The listing builds one solid part. Answer for the finished solid, in the listing's coordinates (mm). Face numbers are marked on the shaded views. A direction names the side the tool comes from. Coordinates: 2 decimals unless noted, no trailing zeros. Write each loop counter-clockwise with the first axis right and the second up, starting at its lowest first coordinate (ties: lowest second). Pieces come first, ordered by that corner, then holes.
from build123d import *

# Parameters (mm, degrees)
F0_R     = 14.2875
F1_DEPTH = 25.4
F2_DEPTH = 50.8


# Not quite as in the source:
# - a fillet or chamfer that OpenCascade refuses, or shapes differently, is made with other operations: its cross-section is extruded or revolved along the edge and cut away or added


with BuildPart() as f1:
    # F0 (on Top) → F1 (new body)
    with BuildSketch(Plane.XY):
        with BuildLine():
            ThreePointArc((5.0426470588, -28.1265414802), (21.9160245563, -18.3362616868), (28.575, 0))
            ThreePointArc((28.575, 0), (21.9160245563, 18.3362616868), (5.0426470588, 28.1265414802))
            ThreePointArc((5.0426470588, 28.1265414802), (-28.575, 0), (5.0426470588, -28.1265414802))
        make_face()
        with BuildLine():
            ThreePointArc((-13.4703841816, 4.7625), (0, 14.2875), (13.4703841816, 4.7625))
            Line((13.4703841816, 4.7625), (19.05, 4.7625))
            Line((19.05, 4.7625), (19.05, -4.7625))
            Line((19.05, -4.7625), (13.4703841816, -4.7625))
            ThreePointArc((13.4703841816, -4.7625), (0, -14.2875), (-13.4703841816, -4.7625))
            Line((-13.4703841816, -4.7625), (-19.05, -4.7625))
            Line((-19.05, -4.7625), (-19.05, 4.7625))
            Line((-19.05, 4.7625), (-13.4703841816, 4.7625))
        make_face(mode=Mode.SUBTRACT)
        with BuildLine():
            ThreePointArc((5.0426470588, 28.1265414802), (21.9160245563, 18.3362616868), (28.575, 0))
            ThreePointArc((28.575, 0), (21.9160245563, -18.3362616868), (5.0426470588, -28.1265414802))
            Line((5.0426470588, -28.1265414802), (57.3367647059, -18.7510276535))
            ThreePointArc((57.3367647059, -18.7510276535), (34.925, 0), (57.3367647059, 18.7510276535))
            Line((57.3367647059, 18.7510276535), (5.0426470588, 28.1265414802))
        make_face()
        with BuildLine():
            ThreePointArc((-13.4703841816, -4.7625), (-14.2875, 0), (-13.4703841816, 4.7625))
            Line((-13.4703841816, 4.7625), (-19.05, 4.7625))
            Line((-19.05, 4.7625), (-19.05, -4.7625))
            Line((-19.05, -4.7625), (-13.4703841816, -4.7625))
        make_face()
        with BuildLine():
            ThreePointArc((73.025, 0), (68.5856830375, 12.2241744579), (57.3367647059, 18.7510276535))
            ThreePointArc((57.3367647059, 18.7510276535), (34.925, 0), (57.3367647059, -18.7510276535))
            ThreePointArc((57.3367647059, -18.7510276535), (68.5856830375, -12.2241744579), (73.025, 0))
        make_face()
        with Locations((53.975, 0)):
            Circle(F0_R, mode=Mode.SUBTRACT)
    extrude(amount=F1_DEPTH)

    # F0 (on Top) → F2 (join)
    with BuildSketch(Plane.XY):
        with BuildLine():
            ThreePointArc((5.0426470588, -28.1265414802), (21.9160245563, -18.3362616868), (28.575, 0))
            ThreePointArc((28.575, 0), (21.9160245563, 18.3362616868), (5.0426470588, 28.1265414802))
            ThreePointArc((5.0426470588, 28.1265414802), (-28.575, 0), (5.0426470588, -28.1265414802))
        make_face()
        with BuildLine():
            ThreePointArc((-13.4703841816, 4.7625), (0, 14.2875), (13.4703841816, 4.7625))
            Line((13.4703841816, 4.7625), (19.05, 4.7625))
            Line((19.05, 4.7625), (19.05, -4.7625))
            Line((19.05, -4.7625), (13.4703841816, -4.7625))
            ThreePointArc((13.4703841816, -4.7625), (0, -14.2875), (-13.4703841816, -4.7625))
            Line((-13.4703841816, -4.7625), (-19.05, -4.7625))
            Line((-19.05, -4.7625), (-19.05, 4.7625))
            Line((-19.05, 4.7625), (-13.4703841816, 4.7625))
        make_face(mode=Mode.SUBTRACT)
        with BuildLine():
            ThreePointArc((-13.4703841816, -4.7625), (-14.2875, 0), (-13.4703841816, 4.7625))
            Line((-13.4703841816, 4.7625), (-19.05, 4.7625))
            Line((-19.05, 4.7625), (-19.05, -4.7625))
            Line((-19.05, -4.7625), (-13.4703841816, -4.7625))
        make_face()
    extrude(amount=F2_DEPTH)

    # F3: fillet of radius 17.78 on 1 edges, made by hand

    # F3_s1 → F3_t2 (revolve, cut)
    with BuildSketch(Plane(origin=(0, 0, 0), x_dir=(0, 0, 1), z_dir=(-0.9843059136, -0.1764705882, 0))):
        with BuildLine():
            ThreePointArc((33.02, -28.575), (45.5923585695, -23.3673585695), (50.8, -10.795))
            Line((50.8, -10.795), (50.8, -28.575))
            Line((50.8, -28.575), (33.02, -28.575))
        make_face()
    revolve(axis=Axis((0, 0, 50.8), (0, 0, 1)), mode=Mode.SUBTRACT)


solid = f1.part
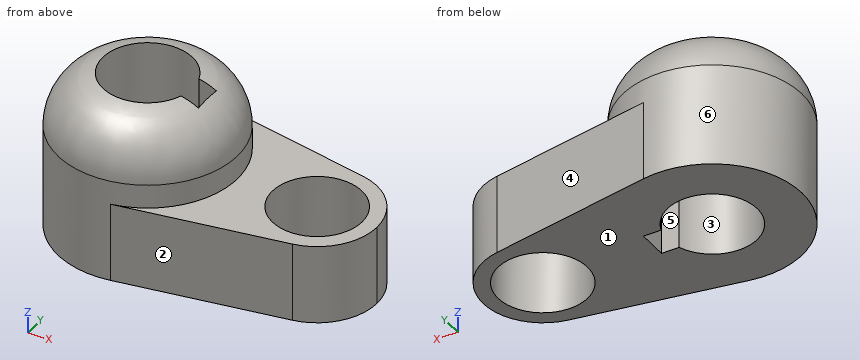
Q1. Which of the six approach directions +Z, -Z, +X, -X, +Y, -Y give full straight-line access (tool end or side, diameter ignored) to the marked faces 4, 5 and 6?
Answers below:
face 4: +Z, -Z, +X, +Y
face 5: +Z, -Z
face 6: +Z
Q2. Find the intervals of material crossed by probe 1 along X at (y, z) = (6, 6.5); probe 2 along Y at (x, z) = (0, 29) (1 decimal); probe 3 along X at (y, z) = (-1, 16), in increasing order.
Answers below:
probe 1: x = -27.94 to -12.97, 12.97 to 41.01, 66.94 to 72.06
probe 2: y = -28.6 to -14.3, 14.3 to 28.6
probe 3: x = -28.56 to -14.25, 19.05 to 39.72, 68.23 to 73
Q3. The part is cut by section B-B, the plane x = 52.5. Write down the section's boundary in (y, z).
Answers below:
outline: (-19.62, 0) - (-14.21, 0) - (-14.21, 25.4) - (-19.62, 25.4) - close; (14.21, 0) - (19.62, 0) - (19.62, 25.4) - (14.21, 25.4) - close
Q4. Given pin 1 (8 mm diameter, centred on x = 12, y = 17.5, fed in from +Z); pin 2 (10 mm diameter, centred on y = -9, z = 39, fed in from +X); pin 3 (1.5 mm diameter, centred on y = 11, z = 33.5, fed in from -X), each flat-ended and moving along its own axis, determine where each tip first touches the part or whether it passes through.
Answers below:
pin 1: stops at z = 49.6
pin 2: stops at x = 27.88
pin 3: stops at x = -26.67
Q5. The part is cut by section A-A, the plane z = 20. State how many separate pieces and enclosed holes the cut face has, then the cut area to 3 significant figures.
Answers below:
separate pieces: 1
enclosed holes: 2
area: 3,130 mm2
Q6. Determine the mould class of the marked faces 1, 2 and 3 for opening direction Y: released by +Y, released by -Y, zero draft, split by the parting line, or undercut.
Answers below:
face 1: zero draft
face 2: released by -Y
face 3: undercut
